```python
from build123d import *

# Parameters (mm, degrees)
PAD072_DEPTH            = 2
CYLINDER084_R           = 2.2
CYLINDER084_DEPTH       = 7
SKETCH123_R             = 1.4
POCKET026_DEPTH         = 7.401
CHAMFER001_SIZE         = 1.5
BODY090_PLACEMENT_ANGLE = 180
BODY093_ROLL_ANGLE      = 90
BODY093_PLACEMENT_ANGLE = 180


with BuildPart() as part:
    # Sketch122 → Pad072 (new body)
    with BuildSketch(Plane.XZ):
        with BuildLine():
            Line((-4, -2.5), (-19.6, -2.5))
            Line((-19.6, -2.5), (-19.6, -10.5))
            Line((-19.6, -10.5), (19.6, -10.5))
            Line((19.6, -10.5), (19.6, -2.5))
            Line((19.6, -2.5), (4, -2.5))
            ThreePointArc((4, -2.5), (0, 1.5), (-4, -2.5))
        make_face()
        with BuildLine():
            ThreePointArc((1.7, -2), (0, -0.3), (-1.7, -2))
            Line((-1.7, -2), (-1.7, -3))
            ThreePointArc((-1.7, -3), (0, -4.7), (1.7, -3))
            Line((1.7, -3), (1.7, -2))
        make_face(mode=Mode.SUBTRACT)
    extrude(amount=PAD072_DEPTH)

    # Cylinder084 → Cylinder084 (join)
    with BuildSketch(Plane(origin=(7.25, 5.4, -6.5), x_dir=(1, 0, 0), z_dir=(0, -1, 0))):
        Circle(CYLINDER084_R)
    cylinder084 = extrude(amount=CYLINDER084_DEPTH)

    # Mirrored020: Cylinder084 across YZ
    add(cylinder084.mirror(Plane.YZ))

    # Sketch123 → Pocket026 (cut, through all)
    with BuildSketch(Plane.XZ.offset(2)):
        with Locations((-7.25, -6.5)):
            Circle(SKETCH123_R)
        with Locations((7.25, -6.5)):
            Circle(SKETCH123_R)
    extrude(amount=-POCKET026_DEPTH, mode=Mode.SUBTRACT)

    # Chamfer001
    chamfer001_edges = [part.edges().sort_by_distance(p)[0] for p in [
        (-8.65, -2, -6.5),
        (5.85, -2, -6.5),
    ]]
    chamfer(chamfer001_edges, length=CHAMFER001_SIZE)


with BuildPart() as part_1:
    # Body090 placement: moved
    add(part.part.moved(Location((0, 4.2, 0))).rotate(Axis((0, 4.2, 0), (0, 0, 1)), BODY090_PLACEMENT_ANGLE))


with BuildPart() as part_2:
    # Clone023 placement: moved
    add(part_1.part.moved(Location((0, -4.2, 0))))


with BuildPart() as part_3:
    # Body093 roll: moved
    add(part_2.part.rotate(Axis((0, 0, 0), (1, 0, 0)), BODY093_ROLL_ANGLE))


with BuildPart() as part_4:
    # Body093 placement: moved
    add(part_3.part.moved(Location((40, 17, 58.2))).rotate(Axis((40, 17, 58.2), (0, 0, 1)), BODY093_PLACEMENT_ANGLE))


solid = part_4.part
```
CAD build for the part. Positions are in the model's coordinates, mm. A direction names the side the tool comes from. Round coordinates to 2 decimals unless told otherwise and drop trailing zeros. Order: outer loops, then holes, each group sorted by start corner. A loop starts at its lowest first (then second) coordinate and runs counter-clockwise, first axis right, second up.
Q1. Slice it at C-C (x = 47.25). Write the cut outline in (y, z), and give its area (3 significant figures).
Q2. Slice it at A-A (x = 40). Write the cut outline in (y, z), and give its area (3 significant figures).
Q3. Which spindle directions (+Z, -Z, +X, -X, +Y, -Y) get a long thin tool onto all of the face, cutting with end or side? Do faces 1 (the flat face through (52, 14.5, 59)), 2 (the flat face through (38.3, 14.5, 59.2)), 3 (the cylindrical face through (45.052, 10.597, 55.462)), 4 (the flat face through (28, 14.5, 59)). Say none if no direction does.
Q4. Drop flat-ended pins along their axis: pin 1 (1.7 mm diameter, centred on x = 32.75, y = 10.5, fed in from -Z); pin 2 (2 mm diameter, centred on x = 33, y = 14.5, fed in from -Z); pin 3 (0.6 mm diameter, centred on x = 53, z = 59, fed in from +Y). Give the stop position or say it passes through.
Q5. Wall check: L1, parallel to X at y = 11.25, z = 53; L2, parallel to Y at x = 32.75, z = 57.3; L3, parallel to X at y = 12.25, z = 59.25. Give the ranges that are in metal, low to high.
Q6. Two-plate mould, pull along Y, no slides. Class faces 5 (the flat face through (41.7, 14.5, 59.2)), 6 (the cylindrical face through (40.1, 18.5, 59.2)), 7 (the cylindrical face through (34.37, 11.99, 55.46)): pulls with the +Y half, pulls with the -Y half, needs draft (parallel to the pull), parting line crosses it, or undercut.
Q7. Slice it at D-D (x = 28). Write the cut outline in (y, z).
Q8. Slice it at B-B (z = 56.25). Write the cut outline in (x, y), and give its area (3 significant figures).
Results below:
1. outline: (6.5, 58.2) - (8.3, 58.2) - (8.3, 52.8) - (9.1, 52.8) - (9.1, 58.7) - (7.6, 60.2) - (6.5, 60.2) - close; (11.9, 52.8) - (12.7, 52.8) - (12.7, 58.2) - (14.5, 58.2) - (14.5, 60.2) - (13.4, 60.2) - (11.9, 58.7) - close
1. area: 16.8 mm2
2. outline: (6.5, 58.2) - (12.3, 58.2) - (12.3, 60.2) - (6.5, 60.2) - close; (16.7, 58.2) - (18.5, 58.2) - (18.5, 60.2) - (16.7, 60.2) - close
2. area: 15.2 mm2
3. face 1: +Z, -Z, +X, +Y
3. face 2: +Z, -Z
3. face 3: -Z
3. face 4: +Z, -Z, -X, +Y
4. pin 1: passes through
4. pin 2: stops at z = 58.2
4. pin 3: stops at y = 14.5
5. L1: x = 30.68 to 31.57, 33.93 to 34.82, 45.18 to 46.07, 48.43 to 49.32
5. L2: y = 8.3 to 9.1, 11.9 to 12.7
5. L3: x = 20.4 to 31.89, 33.61 to 46.39, 48.11 to 59.6
6. face 5: undercut
6. face 6: pulls with the +Y half
6. face 7: parting line crosses it
7. outline: (6.5, 58.2) - (14.5, 58.2) - (14.5, 60.2) - (6.5, 60.2) - close
8. outline: circle Ø4.4 at (32.75, 10.5); circle Ø4.4 at (47.25, 10.5); hole circle Ø2.8 at (32.75, 10.5); hole circle Ø2.8 at (47.25, 10.5)
8. area: 18.1 mm2
